CAD build for the part. Positions are in the model's coordinates, mm. A direction names the side the tool comes from. Coordinates: 2 decimals unless noted, no trailing zeros. Loops run counter-clockwise (first coordinate to the right, second up) from the corner with the lowest first, then second, coordinate; pieces in that order, holes last. Notation, with made-up numbers: (-8, 3) -> (40, 3) arc R25 cw to (40, 31) -> close; hole circle Ø7 at (5, 13). An arc over 180 degrees is marked (long way). Return JSON: item names as keys, results as strings. Group by question number.
(1) Tool access for faces 1 (the face through (-102, 0, -2)), 2 (the face through (-105, -16.089, 9)), 3 (the face through (-2.17, -9.76, 8.87)): list every direction of +Z, -Z, +X, -X, +Y, -Y with a clear straight run to the whole face (end or side of a thin tool).
(2) Saw through at D-D on z = 11.5. Write the cut outline in (x, y), then the cut area to 3 significant figures.
(3) Saw through at C-C on y = 0. Write the cut outline in (x, z), then the cut area to 3 significant figures.
(4) Flat gauge pins, fed straight in: pin 1 Ø10 at (x, z) = (-42, 19.5) entering from +Y; pin 2 Ø2.5 at (y, z) = (-6.5, 19.5) entering from +X; pin 3 Ø5 at (y, z) = (7, -2) entering from -X; pin 4 Ø13 at (x, y) = (-130, 0) entering from +Z. Where does each tip first touch, or does it go through?
(5) Saw through at A-A on z = -2.5. Write the cut outline in (x, y).
(6) Probe L1, parallel to X at y = 174, z = 1; L2, parallel to X at y = -2, z = 20.25; L3, parallel to Z at x = -52, y = 8. List the from-to ranges inside material, lowest first.
(7) Saw through at B-B on x = -130. Write the cut outline in (y, z).
(8) Mould opens along Z. For faces 4 (the face through (1, 46, 0)), 5 (the face through (-108, 0, 9)), 6 (the face through (47.576, 79.464, 8.874)), 7 (the face through (-120, 0, 17)) say: pulls with the +Z half, pulls with the -Z half, needs draft (parallel to the pull), parting line crosses it, or undercut.
```python
from build123d import *

# Parameters (mm, degrees)
EXTRUDE_1_DEPTH     = 18
SKETCH_2_R          = 4
SKETCH_2_R_2        = 10
CUT_EXTRUDE_1_DEPTH = 18
SKETCH_4_W          = 33.000030669
SKETCH_4_H          = 62.878436815
CUT_EXTRUDE_2_DEPTH = 60
EXTRUDE_2_DEPTH     = 6
EXTRUDE_START       = -5
EXTRUDE_3_DEPTH     = 6
EXTRUDE_START_2     = 17
EXTRUDE_4_DEPTH     = 6
SKETCH_7_R          = 4
CUT_EXTRUDE_3_DEPTH = 30


with BuildPart() as part:
    # 草图1 → 凸台-拉伸1 (new body)
    with BuildSketch(Plane.XY):
        with BuildLine():
            Line((48.810330778, 177.946063765), (-10.210076964, 28.583512616))
            ThreePointArc((-10.210076964, 28.583512616), (-15.488001892, 21.85715805), (-23.583519409, 19.107079247))
            Line((-23.583519409, 19.107079247), (-130.576923077, 14.988901219))
            ThreePointArc((-130.576923077, 14.988901219), (-145, 0), (-130.576923077, -14.988901219))
            Line((-130.576923077, -14.988901219), (-0.769230769, -19.985201626))
            ThreePointArc((-0.769230769, -19.985201626), (11.379442316, -16.447136303), (18.973261361, -6.325768991))
            Line((18.973261361, -6.325768991), (76.990642321, 167.689269171))
            ThreePointArc((76.990642321, 167.689269171), (67.89099845, 186.528985226), (48.810330778, 177.946063765))
        make_face()
    extrude(amount=EXTRUDE_1_DEPTH)

    # 草图2 → 切除-拉伸1 (cut)
    with BuildSketch(Plane.XY):
        with Locations((62.7606963, 172.433595914)):
            Circle(SKETCH_2_R)
        Circle(SKETCH_2_R_2)
    extrude(amount=CUT_EXTRUDE_1_DEPTH, mode=Mode.SUBTRACT)

    # 草图4 → 切除-拉伸2 (cut)
    with BuildSketch(Plane.ZY.offset(102)):
        with Locations((8.194839776, -6.074779021)):
            Rectangle(SKETCH_4_W, SKETCH_4_H)
    extrude(amount=CUT_EXTRUDE_2_DEPTH, mode=Mode.SUBTRACT)

    # 草图5 → 凸台-拉伸2 (add)
    with BuildSketch(Plane.ZY.offset(102)):
        Polygon((9, -16.088827501), (-5, -16.088827501), (-5, 16.088827501), (9, 16.088827501), (23, 16.088827501), (23, -16.088827501), align=None)
    extrude(amount=EXTRUDE_2_DEPTH)

    # 草图6 → 凸台-拉伸3 (add)
    with BuildSketch(Plane.XY.offset(EXTRUDE_START)):
        with BuildLine():
            Line((-108, 16.088827501), (-132.619002915, 7.559282635))
            ThreePointArc((-132.619002915, 7.559282635), (-138.000120638, 0), (-132.619002915, -7.559282635))
            Line((-132.619002915, -7.559282635), (-108, -16.088827501))
            Line((-108, -16.088827501), (-108, 16.088827501))
        make_face()
    extrude(amount=EXTRUDE_3_DEPTH)

    # 草图6<2> → 凸台-拉伸4 (add)
    with BuildSketch(Plane.XY.offset(EXTRUDE_START_2)):
        with BuildLine():
            Line((-108, 16.088827501), (-132.619002915, 7.559282635))
            ThreePointArc((-132.619002915, 7.559282635), (-138.000120638, 0), (-132.619002915, -7.559282635))
            Line((-132.619002915, -7.559282635), (-108, -16.088827501))
            Line((-108, -16.088827501), (-108, 16.088827501))
        make_face()
    extrude(amount=EXTRUDE_4_DEPTH)

    # 草图7 → 切除-拉伸3 (cut, symmetric)
    with BuildSketch(Plane.XY):
        with Locations((-130, 0)):
            Circle(SKETCH_7_R)
    extrude(amount=CUT_EXTRUDE_3_DEPTH, both=True, mode=Mode.SUBTRACT)


solid = part.part
```
Geometry results:
{
 "1": {"face 1": "-Z, +X, +Y, -Y", "face 2": "+Z, -Z, -X, -Y", "face 3": "+Z, -Z"},
 "2": {"outline": "(-108, -16.09) -> (-102, -16.09) -> (-0.77, -19.99) arc R20 ccw to (18.97, -6.33) -> (76.99, 167.69) arc R15 ccw to (48.81, 177.95) -> (-10.21, 28.58) arc R15 cw to (-23.58, 19.11) -> (-102, 16.09) -> (-108, 16.09) -> close; hole circle Ø20 at (0, 0); hole circle Ø8 at (62.76, 172.43)", "area": "10,300 mm²"},
 "3": {"outline": "(-138, -5) -> (-134, -5) -> (-134, 1) -> (-138, 1) -> close; (-138, 17) -> (-134, 17) -> (-134, 23) -> (-138, 23) -> close; (-126, -5) -> (-102, -5) -> (-102, 0) -> (-10, 0) -> (-10, 18) -> (-102, 18) -> (-102, 23) -> (-126, 23) -> (-126, 17) -> (-108, 17) -> (-108, 1) -> (-126, 1) -> close; (10, 0) -> (21.08, 0) -> (21.08, 18) -> (10, 18) -> close", "area": "2,290 mm²"},
 "4": {"pin 1": "y = 18.58", "pin 2": "x = -102", "pin 3": "x = -136.61", "pin 4": "z = 23"},
 "5": {"outline": "(-132.62, -7.56) -> (-108, -16.09) -> (-102, -16.09) -> (-102, 16.09) -> (-108, 16.09) -> (-132.62, 7.56) arc R8 ccw to start; hole circle Ø8 at (-130, 0)"},
 "6": {"L1": "47.25 to 59.08, 66.44 to 77.68", "L2": "-137.75 to -133.46, -126.54 to -102", "L3": "0 to 18"},
 "7": {"outline": "(-8.47, -5) -> (-4, -5) -> (-4, 1) -> (-8.47, 1) -> close; (-8.47, 17) -> (-4, 17) -> (-4, 23) -> (-8.47, 23) -> close; (4, -5) -> (8.47, -5) -> (8.47, 1) -> (4, 1) -> close; (4, 17) -> (8.47, 17) -> (8.47, 23) -> (4, 23) -> close"},
 "8": {"face 4": "pulls with the -Z half", "face 5": "undercut", "face 6": "needs draft", "face 7": "undercut"}
}
